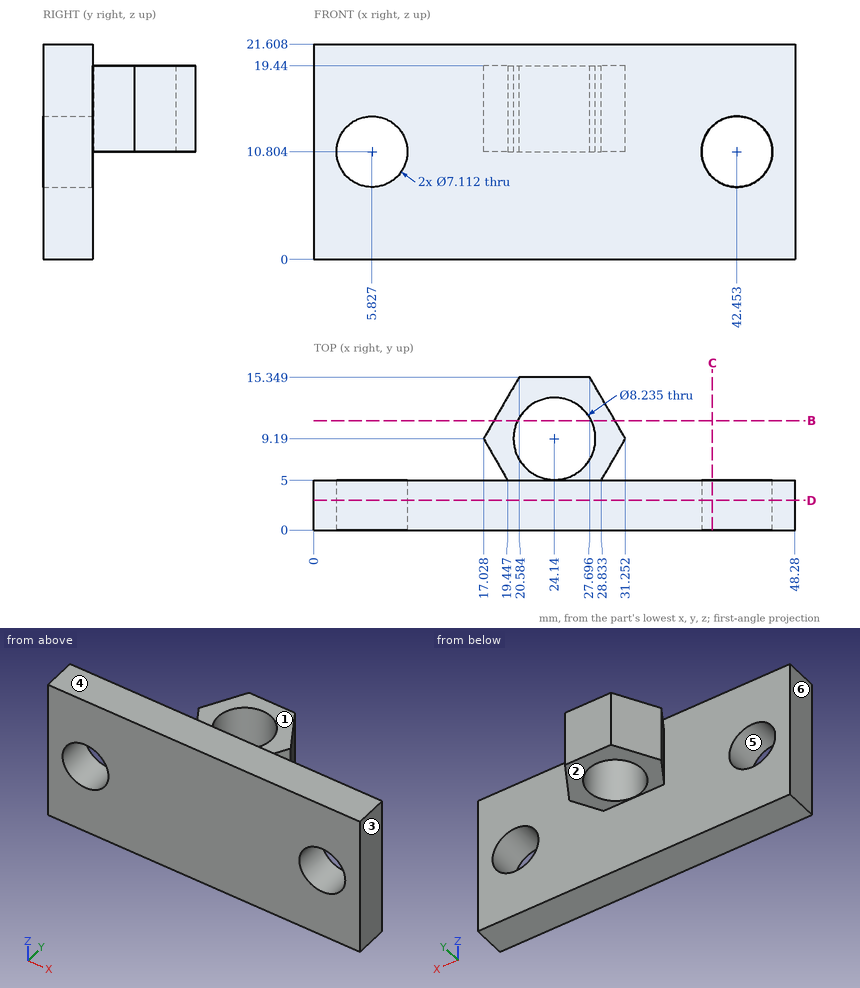
Geometry check sheet. Reference: drawing and pictorial views, mm from the part's lowest x, y, z. A direction names the side the tool comes from. Coordinates: 2 decimals unless noted, no trailing zeros. Order: outer loops, then holes, each group sorted by start corner. A loop starts at its lowest first (then second) coordinate and runs counter-clockwise, first axis right, second up.
Item 1: Access from +Z, -Z, +X, -X, +Y, -Y to the whole of each face (thin tool, end or side, straight path). Record for the marked faces 1, 2 and 3.
Filled in:
face 1: +Z, +X, -X, +Y
face 2: -Z, +X, -X, +Y
face 3: +Z, -Z, +X, +Y, -Y
Item 2: Section check D-D, the plane y = 3. Enter the section's corners in (x, z).
Filled in:
outline: (0, 0) - (48.28, 0) - (48.28, 21.61) - (0, 21.61) - close; hole circle Ø7.11 at (5.83, 10.8); hole circle Ø7.11 at (42.45, 10.8)
Item 3: Material ranges on L1, parallel to X at y = 4.75, z = 11.75 (1 decimal); L2, parallel to Y at x = 22.5, z = 4; L3, parallel to X at y = 2.25, z = 8.5 (1 decimal), recorded low to high.
Filled in:
L1: x = 0 to 2.4, 9.3 to 39, 45.9 to 48.3
L2: y = 0 to 5
L3: x = 0 to 3.1, 8.5 to 39.7, 45.2 to 48.3
Item 4: Section check B-B, the plane y = 11. Enter the section's corners in (x, z).
Filled in:
outline: (18.07, 10.8) - (20.44, 10.8) - (20.44, 19.44) - (18.07, 19.44) - close; (27.84, 10.8) - (30.21, 10.8) - (30.21, 19.44) - (27.84, 19.44) - close
Item 5: Depth check by flat-ended pin: pin 1 (2 mm diameter, centred on x = 21, y = 7, fed in from +Z). Enter the tip coordinate at first touch or a pass-through.
Filled in:
pin 1: stops at z = 19.44
Item 6: Section check C-C, the plane x = 40. Enter the section's corners in (y, z).
Filled in:
outline: (0, 0) - (5, 0) - (5, 8.23) - (0, 8.23) - close; (0, 13.38) - (5, 13.38) - (5, 21.61) - (0, 21.61) - close
Item 7: Release check for a two-part mould opening along Z. For the marked faces 4, 5 and 6 record: +Z half, -Z half, draft (parallel to the pull), parting line (faces both ways), or undercut.
Filled in:
face 4: +Z half
face 5: undercut
face 6: draft
